Read the model definition and answer for the solid it produces. Units are mm, in the model's axes. Face numbers are marked on the shaded views. A direction names the side the tool comes from. Coordinates: 2 decimals unless noted, no trailing zeros. Order: outer loops, then holes, each group sorted by start corner. A loop starts at its lowest first (then second) coordinate and runs counter-clockwise, first axis right, second up. Notation, with made-up numbers: M 15.25,-39.75 L 31.25,-39.75 A26 ccw 31.25,-13.75 Z; hole C -31,77.25 d8. An arc over 180 degrees is marked long. Use a Markdown table: item, result. Add a question column.
1) Find section B-B on z = -1. Write down the section's boundary in (x, y).
2) Find section C-C on x = -15.25. Write down the section's boundary in (y, z).
3) Find the intervals of material crossed by probe 1 along Y at (x, z) = (0, 3.6); probe 2 along Y at (x, z) = (0, 2); probe 3 along X at (y, z) = (-7.75, 2.25), in increasing order. Write a range as [from, to].
4) Each of these flat-tipped pins is pushed along its axis until it touches: pin 1 Ø2.5 at (y, z) = (-0.5, -32.5) entering from -X; pin 2 Ø1.8 at (x, y) = (0.5, -1) entering from -Z; pin 3 Ø1.2 at (x, y) = (-13.42, -7.75) entering from +Z; pin 4 Ø3 at (y, z) = (1.5, -0.5) entering from +X. Where does it stop, or does it pass through?
5) The mould has two halves that part along Z. Classify the marked faces 4, 5, 6 and 7: released by +Z, released by -Z, zero draft, split by the parting line, or undercut.
6) Find section A-A on y = 15.5. Write down the section's boundary in (x, z).
7) Find section D-D on x = -8. Write down the section's boundary in (y, z), plus the area to 3 significant figures.
8) For the marked faces 1, 2 and 3, determine the directions among +Z, -Z, +X, -X, +Y, -Y from which every point of the face is accessible in a straight line to the end or side of a thin tool.
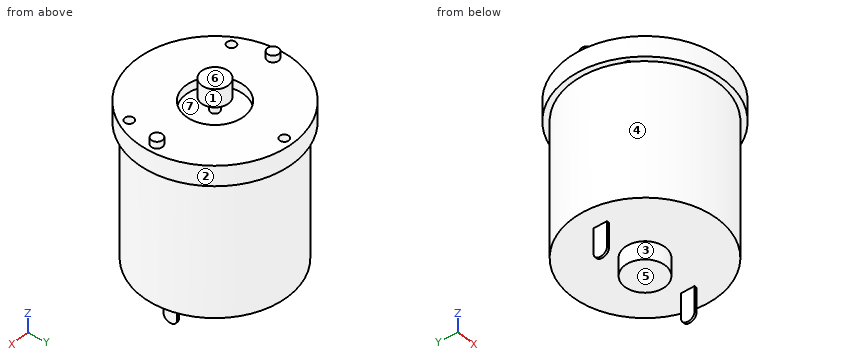
from build123d import *

# Parameters (mm, degrees)
SKETCH_R        = 17.5
PAD_DEPTH       = 4.5
SKETCH001_R     = 16.25
PAD001_DEPTH    = 30
SKETCH002_R     = 4.5
PAD002_DEPTH    = 4
SKETCH003_W     = 0.5
SKETCH003_H     = 3
PAD003_DEPTH    = 7
FILLET_R        = 1.4
SKETCH004_R     = 1.25
PAD004_DEPTH    = 1.5
SKETCH005_R     = 1
POCKET_DEPTH    = 4.5
SKETCH006_R     = 6.5
POCKET001_DEPTH = 2
SKETCH007_R     = 1
PAD005_DEPTH    = 7
SKETCH008_R     = 3
PAD006_DEPTH    = 4


with BuildPart() as part:
    # Sketch → Pad (new body)
    with BuildSketch(Plane.XY):
        Circle(SKETCH_R)
    extrude(amount=PAD_DEPTH)

    # Sketch001 (on Face2 of Pad) → Pad001 (join)
    with BuildSketch(Plane(origin=(0, 0, 0), x_dir=(1, 0, 0), z_dir=(0, 0, -1))):
        Circle(SKETCH001_R)
    extrude(amount=PAD001_DEPTH)

    # Sketch002 (on Face5 of Pad001) → Pad002 (join)
    with BuildSketch(Plane(origin=(0, 0, -30), x_dir=(1, 0, 0), z_dir=(0, 0, -1))):
        Circle(SKETCH002_R)
    extrude(amount=PAD002_DEPTH)

    # Sketch003 (on Face5 of Pad002) → Pad003 (join)
    with BuildSketch(Plane(origin=(0, 0, -30), x_dir=(1, 0, 0), z_dir=(0, 0, -1))):
        with Locations((11.5, 0)):
            Rectangle(SKETCH003_W, SKETCH003_H)
        with Locations((-11.5, 0)):
            Rectangle(SKETCH003_W, SKETCH003_H)
    extrude(amount=PAD003_DEPTH)

    # Fillet
    fillet_edges = [part.edges().sort_by_distance(p)[0] for p in [
        (11.5, -1.5, -37),
        (11.5, 1.5, -37),
        (-11.5, 1.5, -37),
        (-11.5, -1.5, -37),
    ]]
    fillet(fillet_edges, radius=FILLET_R)

    # Sketch004 (on Face21 of Fillet) → Pad004 (join)
    with BuildSketch(Plane.XY.offset(4.5)):
        with Locations((-15.25, 0)):
            Circle(SKETCH004_R)
        with Locations((15.25, 0)):
            Circle(SKETCH004_R)
    extrude(amount=PAD004_DEPTH)

    # Sketch005 (on Face21 of Pad004) → Pocket (cut)
    with BuildSketch(Plane.XY.offset(4.5)):
        with Locations((0, 15.5)):
            Circle(SKETCH005_R)
        with Locations((-13.423394, -7.75)):
            Circle(SKETCH005_R)
        with Locations((13.423394, -7.75)):
            Circle(SKETCH005_R)
    extrude(amount=-POCKET_DEPTH, mode=Mode.SUBTRACT)

    # Sketch006 (on Face27 of Pocket) → Pocket001 (cut)
    with BuildSketch(Plane.XY.offset(4.5)):
        Circle(SKETCH006_R)
    extrude(amount=-POCKET001_DEPTH, mode=Mode.SUBTRACT)

    # Sketch007 (on Face32 of Pocket001) → Pad005 (join)
    with BuildSketch(Plane.XY.offset(2.5)):
        Circle(SKETCH007_R)
    extrude(amount=PAD005_DEPTH)

    # Sketch008 (on Face35 of Pad005) → Pad006 (join)
    with BuildSketch(Plane.XY.offset(9.5)):
        Circle(SKETCH008_R)
    extrude(amount=-PAD006_DEPTH)


solid = part.part
Check result:
| question | item | result |
|---|---|---|
| 1 | outline | C 0,0 d32.5 |
| 2 | outline | M -8.58,0 L -5.61,0 L -5.61,-30 L 5.61,-30 L 5.61,0 L 8.58,0 L 8.58,4.5 L 1.25,4.5 L 1.25,6 L -1.25,6 L -1.25,4.5 L -8.58,4.5 Z |
| 3 | probe 1 | y = [-17.5, -6.5], [-1, 1], [6.5, 14.5], [16.5, 17.5] |
| 3 | probe 2 | y = [-17.5, 14.5], [16.5, 17.5] |
| 3 | probe 3 | x = [-15.69, -14.42], [-12.42, 12.42], [14.42, 15.69] |
| 4 | pin 1 | stops at x = -11.75 |
| 4 | pin 2 | stops at z = -34 |
| 4 | pin 3 | stops at z = 0 |
| 4 | pin 4 | stops at x = 17.5 |
| 5 | face 4 | zero draft |
| 5 | face 5 | released by -Z |
| 5 | face 6 | released by +Z |
| 5 | face 7 | undercut |
| 6 | outline | M -8.12,0 L -4.88,0 L -4.88,-30 L 4.88,-30 L 4.88,0 L 8.12,0 L 8.12,4.5 L 1,4.5 L 1,0 L -1,0 L -1,4.5 L -8.12,4.5 Z |
| 7 | outline | M -15.56,0 L -14.14,0 L -14.14,-30 L 14.14,-30 L 14.14,0 L 15.56,0 L 15.56,4.5 L -15.56,4.5 Z |
| 7 | area | 989 mm2 |
| 8 | face 1 | +Z |
| 8 | face 2 | +Z, -Z |
| 8 | face 3 | -Z |
